from build123d import *

# Parameters (mm, degrees)
BOSS_EXTRUDE1_DEPTH     = 51.000025
SKETCH5_R               = 0.55245
CUT_EXTRUDE1_DEPTH      = 52.000025
CUT_EXTRUDE1_DEPTH_BACK = 52.000025


with BuildPart() as part:
    # Sketch4 → Boss-Extrude1 (new body, symmetric)
    with BuildSketch(Plane.XY):
        with BuildLine():
            Line((4.190365, -12.7), (10.11729625, -12.7))
            ThreePointArc((10.11729625, -12.7), (11.943543585, -11.943543585), (12.7, -10.11729625))
            Line((12.7, -10.11729625), (12.7, -4.190365))
            ThreePointArc((12.7, -4.190365), (12.42492494, -3.52627506), (11.760835, -3.2512))
            Line((11.760835, -3.2512), (11.429365, -3.2512))
            ThreePointArc((11.429365, -3.2512), (10.76527506, -3.52627506), (10.4902, -4.190365))
            Line((10.4902, -4.190365), (10.4902, -6.348478019))
            ThreePointArc((10.4902, -6.348478019), (9.830707141, -7.335478831), (8.666460301, -7.103895736))
            Line((8.666460301, -7.103895736), (5.299899128, -3.737334563))
            ThreePointArc((5.299899128, -3.737334563), (4.817571085, -3.015479634), (4.6482, -2.16399369))
            Line((4.6482, -2.16399369), (4.6482, 0))
            Line((4.6482, 0), (2.6035, 0))
            ThreePointArc((2.6035, 0), (1.840952505, -1.840952505), (0, -2.6035))
            Line((0, -2.6035), (0, -4.6482))
            Line((0, -4.6482), (2.16399369, -4.6482))
            ThreePointArc((2.16399369, -4.6482), (3.015479634, -4.817571085), (3.737334563, -5.299899128))
            Line((3.737334563, -5.299899128), (7.103895736, -8.666460301))
            ThreePointArc((7.103895736, -8.666460301), (7.335478831, -9.830707141), (6.348478019, -10.4902))
            Line((6.348478019, -10.4902), (4.190365, -10.4902))
            ThreePointArc((4.190365, -10.4902), (3.52627506, -10.76527506), (3.2512, -11.429365))
            Line((3.2512, -11.429365), (3.2512, -11.760835))
            ThreePointArc((3.2512, -11.760835), (3.52627506, -12.42492494), (4.190365, -12.7))
        make_face()
    extrude(amount=BOSS_EXTRUDE1_DEPTH, both=True)

    # Sketch5 → Cut-Extrude1 (cut, two sides)
    with BuildSketch(Plane.XY) as cut_extrude1_sk:
        with Locations((10.356153152, -12.7)):
            Circle(SKETCH5_R)
        with Locations((5.796028019, -12.7)):
            Circle(SKETCH5_R)
        with Locations((12.7, -10.356153152)):
            Circle(SKETCH5_R)
        with Locations((12.7, -5.796028019)):
            Circle(SKETCH5_R)
    extrude(amount=CUT_EXTRUDE1_DEPTH, mode=Mode.SUBTRACT)
    extrude(cut_extrude1_sk.sketch, amount=-CUT_EXTRUDE1_DEPTH_BACK, mode=Mode.SUBTRACT)

    # Mirror1: part across plane


with BuildPart() as part_1:
    add(part.part)
    add(part.part.mirror(Plane(origin=(0, 0, 0), x_dir=(0, 0, 1), z_dir=(1, 0, 0))))

    # Mirror2: part across plane


with BuildPart() as part_2:
    add(part_1.part)
    add(part_1.part.mirror(Plane.ZX))


solid = part_2.part
Geometry check sheet. Reference: the model listing, model coordinates, mm. A direction names the side the tool comes from. Round coordinates to 2 decimals unless told otherwise and drop trailing zeros.
Item 1: Thickness scan on line 1 (X direction, y = -9.25, z = 33); line 2 (Y direction, x = 7, z = -7); line 3 (Y direction, x = -5.75, z = -7). Record the ranges inside material, lowest first.
Item 2: Mould release check, pull along Y, two halves, no side actions. Record for faces 5 (the flat face through (8, 12.7, 1)), 6 (the flat face through (-12.7, 8, 1)), 7 (the cylindrical face through (-9.847, 7.329, 0.714)): pulls with the +Y half, pulls with the -Y half, needs draft (parallel to the pull), parting line crosses it, or undercut.
Item 3: Gauge pin test, flat ends, axial feed: pin 1 (3.5 mm diameter, centred on x = 0, z = 4, fed in from +Y); pin 2 (1.3 mm diameter, centred on y = -1, z = 21.5, fed in from -X); pin 3 (3.5 mm diameter, centred on x = 0, z = 15.5, fed in from -Y); pin 4 (4 mm diameter, centred on x = -9, y = 2, fed in from +Z). Record the tip position at first contact, or that the pin passes through.
Item 4: Access from +Z, -Z, +X, -X, +Y, -Y to the whole of each face (thin tool, end or side, straight path). Record for faces 1 (the flat face through (-8, -12.7, 1)), 2 (the flat face through (0, 4.648, 1)), 3 (the flat face through (5.4, 6.96, 0.71)), 4 (the flat face through (4.648, 0, 1)).
Answer sheet:
1. line 1: x = -12.7 to -7.4, 7.4 to 12.7
1. line 2: y = -12.7 to -10.27, -8.56 to -5.44, 5.44 to 8.56, 10.27 to 12.7
1. line 3: y = -12.15 to -10.49, -7.31 to -4.19, 4.19 to 7.31, 10.49 to 12.15
2. face 5: pulls with the +Y half
2. face 6: needs draft
2. face 7: undercut
3. pin 1: stops at y = 4.65
3. pin 2: stops at x = -4.65
3. pin 3: stops at y = -4.65
3. pin 4: passes through
4. face 1: +Z, -Z, +X, -X, -Y
4. face 2: +Z, -Z, +Y
4. face 3: +Z, -Z
4. face 4: +Z, -Z, +X
